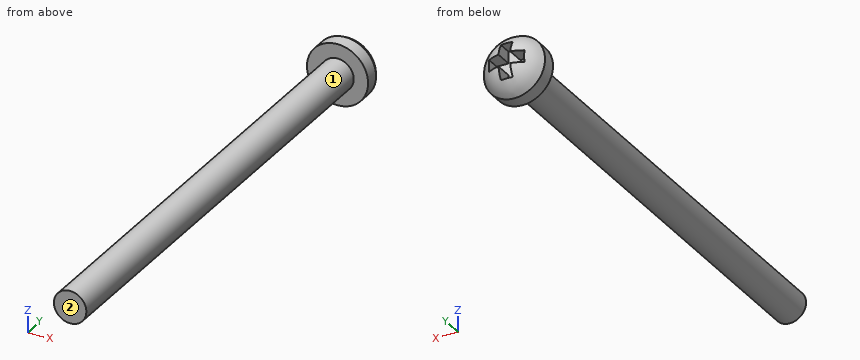
from build123d import *

# Parameters (mm, degrees)
CUT_EXTRUDE1_REACH      = 54.532
CUT_EXTRUDE1_END_RADIUS = 3.68985638


with BuildPart() as part:
    # Sketch1 → Revolve1 (revolve)
    with BuildSketch(Plane.XY, mode=Mode.PRIVATE) as revolve1_sk:
        Polygon((0, 50.677234653), (0, 0), (1.7526, 0), (1.7526, 50.8), (0, 50.8), align=None)
        with BuildLine():
            Line((0, 54.367091034), (0, 50.8))
            Line((0, 50.8), (1.7526, 50.8))
            Line((1.7526, 50.8), (3.302, 50.8))
            Line((3.302, 50.8), (3.302, 52.324))
            ThreePointArc((3.302, 52.324), (1.941483001, 53.815017926), (0, 54.367091034))
        make_face()
    revolve(revolve1_sk.sketch.rotate(Axis((0, -8.932338451, 0), (0, 1, 0)), 90), axis=Axis((0, -8.932338451, 0), (0, 1, 0)))

    # Cut-Extrude1: up to this sphere (the profile starts inside it)
    cut_extrude1_end = Location((0, 50.677234653, 0)) * Sphere(CUT_EXTRUDE1_END_RADIUS, mode=Mode.PRIVATE)
    # Sketch2 → Cut-Extrude1 (cut, up to the surface)
    with BuildSketch(Plane(origin=(0, 52.324, 0), x_dir=(-1, 0, 0), z_dir=(0, -1, 0)), mode=Mode.PRIVATE) as cut_extrude1_sk1:
        Polygon((0.635, 0.635), (1.905, 0.635), (1.905, -0.635), (0.635, -0.635), (0.635, -1.905), (-0.635, -1.905), (-0.635, -0.635), (-1.905, -0.635), (-1.905, 0.635), (-0.635, 0.635), (-0.635, 1.905), (0.635, 1.905), align=None)
    cut_extrude1_tool1 = extrude(cut_extrude1_sk1.sketch, amount=-CUT_EXTRUDE1_REACH, mode=Mode.PRIVATE) & cut_extrude1_end
    add(cut_extrude1_tool1.solids().sort_by_distance((0, 52.324, 0))[0], mode=Mode.SUBTRACT)


solid = part.part
For this review, take the finished solid that the model builds, in its own axes (mm). Face numbers are marked on the shaded views. A direction names the side the tool comes from. Round coordinates to 2 decimals unless told otherwise and drop trailing zeros. Order: outer loops, then holes, each group sorted by start corner. A loop starts at its lowest first (then second) coordinate and runs counter-clockwise, first axis right, second up. Notation, with made-up numbers: (30, 73) -> (70, 73) arc R19 ccw to (70, 106) -> close; hole circle Ø6 at (35.5, 64). An arc over 180 degrees is marked (long way). Write item = value, one per line. Start each with the question number.
1) To check wall thickness, follow line 1 (Y direction, x = 0.25, z = -1.5); line 2 (Z direction, x = -3, y = 51.5); line 3 (Z direction, x = 1.75, y = 51). State the ranges of each line that lie inside material, in increasing order. Write a range as from..to.
2) Insertion check: pin 1 (1 mm diameter, centred on x = -0.5, z = -0.5, fed in from -Y); pin 2 (1.4 mm diameter, centred on x = 1.5, y = 53, fed in from -Z); pin 3 (0.6 mm diameter, centred on x = 1.5, y = 53, fed in from +Z); pin 4 (0.6 mm diameter, centred on y = 53, z = -1.5, fed in from +X). Each pin has a flat end and moves straight along its axis. Give the tip position at first contact, or say it passes through.
3) Take a section at C-C on y = 14.5. State the section outline as (x, z) points.
4) Take a section at B-B on z = 0. State the section outline as (x, y) points (3 decimals), plus the area to 3 significant figures.
5) Take a section at A-A on x = 0. State the section outline as (y, z) points (3 decimals).
6) Take a section at D-D on x = -2.5. State the section outline as (y, z) points, plus the area to 3 significant figures.
7) Tool access review of the marked faces 1 and 2: name each direction out of +Z, -Z, +X, -X, +Y, -Y from which nothing blocks a thin tool from reaching the whole face with its end or side.
Verdict:
q1.line_1 = 0..52.32
q1.line_2 = -1.38..1.38
q1.line_3 = -2.8..2.8
q2.pin_1 = 0
q2.pin_2 = -3.06
q2.pin_3 = 2.75
q2.pin_4 = 2.75
q3.outline = circle Ø3.51 at (0, 0)
q4.outline = (-3.302, 50.8) -> (-1.753, 50.8) -> (-1.753, 0) -> (1.753, 0) -> (1.753, 50.8) -> (3.302, 50.8) -> (3.302, 52.324) arc R3.69 ccw to (1.905, 53.837) -> (1.905, 52.324) -> (-1.905, 52.324) -> (-1.905, 53.837) arc R3.69 ccw to (-3.302, 52.324) -> close
q4.area = 191 mm2
q5.outline = (0, -1.753) -> (50.8, -1.753) -> (50.8, -3.302) -> (52.324, -3.302) arc R3.69 ccw to (53.837, -1.905) -> (52.324, -1.905) -> (52.324, 1.905) -> (53.837, 1.905) arc R3.69 ccw to (52.324, 3.302) -> (50.8, 3.302) -> (50.8, 1.753) -> (0, 1.753) -> close
q6.outline = (50.8, -2.16) -> (52.32, -2.16) arc R2.71 ccw to (52.32, 2.16) -> (50.8, 2.16) -> close
q6.area = 9.79 mm2
q7.face_1 = -Y
q7.face_2 = +Z, -Z, +X, -X, -Y
